from build123d import *

# Parameters (mm, degrees)
SKETCH_1_W             = 35.69
SKETCH_1_H             = 89.14
SM_BASE_FLANGE_1_DEPTH = 2.85
OTHER_START            = -17.845
OTHER_1_DEPTH          = 35.69
OTHER_1_2_DEPTH        = 35.69
SKETCH_7_R             = 14.0825
SKETCH_7_R_2           = 1.845
CUT_EXTRUDE_1_DEPTH    = 10
CHAMFER_1_SIZE         = 3
SKETCH_8_R             = 2.795
CUT_EXTRUDE_2_DEPTH    = 10


# Read off the part's stored shape, not the designer's step: Нарисованный сгиб1
# Sheet-metal steps are written as plain solids
with BuildPart() as part:
    # Sketch 1 → Базовая кромка1 (new body)
    with BuildSketch(Plane(origin=(0, 0, 0), x_dir=(1, 0, 0), z_dir=(0, 1, 0))):
        Rectangle(SKETCH_1_W, SKETCH_1_H)
    extrude(amount=-SM_BASE_FLANGE_1_DEPTH)

    # Other 1 outline → Other 1 (cut)
    with BuildSketch(Plane.YZ.offset(OTHER_START)):
        with BuildLine():
            Line((0, -44.57), (0, 6.169199698))
            ThreePointArc((0, 6.169199698), (-2.096002789, 8.605700079), (-2.85, 11.73))
            Line((-2.85, 11.73), (-2.85, -44.57))
            Line((-2.85, -44.57), (0, -44.57))
        make_face()
    extrude(amount=OTHER_1_DEPTH, mode=Mode.SUBTRACT)

    # Other 1 2 outline → Other 1 2 (add)
    with BuildSketch(Plane.YZ.offset(OTHER_START)):
        with BuildLine():
            Line((51.778429927, 7.73), (4, 7.73))
            ThreePointArc((4, 7.73), (1.171572875, 8.901572875), (0, 11.73))
            Line((0, 11.73), (0, 6.169199698))
            ThreePointArc((0, 6.169199698), (1.898688751, 5.210261429), (4, 4.88))
            Line((4, 4.88), (51.778429927, 4.88))
            Line((51.778429927, 4.88), (51.778429927, 7.73))
        make_face()
    extrude(amount=OTHER_1_2_DEPTH)

    # Эскиз7 → Вырез-Вытянуть1 (cut)
    with BuildSketch(Plane.XY.offset(7.73)):
        with Locations((0, 33.778429927)):
            Circle(SKETCH_7_R)
        with Locations((13, 46.778429927)):
            Circle(SKETCH_7_R_2)
        with Locations(Location((-13, 46.778429927, 0), (0, 0, 90))):
            Circle(SKETCH_7_R_2)
        with Locations((-13, 20.778429927)):
            Circle(SKETCH_7_R_2)
        with Locations(Location((13, 20.778429927, 0), (0, 0, 90))):
            Circle(SKETCH_7_R_2)
    extrude(amount=-CUT_EXTRUDE_1_DEPTH, mode=Mode.SUBTRACT)

    # Фаска1
    chamfer_1_edges = [part.edges().sort_by_distance(p)[0] for p in [
        (17.845, -1.425, 44.57),
        (-17.845, -1.425, 44.57),
        (-17.845, 51.778429927, 6.305),
        (17.845, 51.778429927, 6.305),
    ]]
    chamfer(chamfer_1_edges, length=CHAMFER_1_SIZE)

    # Эскиз8 → Вырез-Вытянуть2 (cut)
    with BuildSketch(Plane(origin=(0, 0, 0), x_dir=(1, 0, 0), z_dir=(0, 1, 0))):
        with Locations(Location((-10, -29.57, 0), (0, 0, 270))):
            Circle(SKETCH_8_R)
        with Locations(Location((10, -29.57, 0), (0, 0, 90))):
            Circle(SKETCH_8_R)
    extrude(amount=-CUT_EXTRUDE_2_DEPTH, mode=Mode.SUBTRACT)


solid = part.part
Build history of the part. All positions in model axes, mm. A direction names the side the tool comes from. Round coordinates to 2 decimals unless told otherwise and drop trailing zeros. Write each loop counter-clockwise with the first axis right and the second up, starting at its lowest first coordinate (ties: lowest second). Pieces come first, ordered by that corner, then holes. Notation, with made-up numbers: (13, -16.5) - (33, -16.5) arc R21 ccw to (33, 1.5) - close; hole circle Ø7 at (38.25, 56.25). An arc over 180 degrees is marked (long way). One line per question, with ' | ' between items.
1. Drop a flat-ended pin along its axis: pin 1 Ø2 at (x, y) = (-11, 19) entering from +Z. Give the stop position or say it passes through.
Results are:
pin 1: z = 7.73
2. Band-saw the part on D-D, the plane x = 9. Write the cut outline in (y, z).
Results are:
outline: (-2.85, 11.73) arc R6.85 ccw to (4, 4.88) - (22.95, 4.88) - (22.95, 7.73) - (4, 7.73) arc R4 cw to (0, 11.73) - (0, 26.96) - (-2.85, 26.96) - close; (-2.85, 32.18) - (0, 32.18) - (0, 44.57) - (-2.85, 44.57) - close; (44.61, 4.88) - (51.78, 4.88) - (51.78, 7.73) - (44.61, 7.73) - close
3. Mould opens along X. For faces 3 (the face through (17.845, 11, 7)), 4 (the face through (-12.15, 19.14, 6.32)), 5 (the face through (-16.324, -1.405, 43.091)), 6 (the face through (0, 17, 4.88)) say: released by +X, released by -X, zero draft, split by the parting line, or undercut.
Results are:
face 3: released by +X | face 4: undercut | face 5: released by -X | face 6: zero draft
4. Band-saw the part on A-A, the plane z = 29.57. Write the cut outline in (x, y) (3 decimals).
Results are:
outline: (-17.845, -2.85) - (-12.795, -2.85) - (-12.795, 0) - (-17.845, 0) - close; (-7.205, -2.85) - (7.205, -2.85) - (7.205, 0) - (-7.205, 0) - close; (12.795, -2.85) - (17.845, -2.85) - (17.845, 0) - (12.795, 0) - close
5. Band-saw the part on C-C, the plane y = 32.5. Write the cut outline in (x, z) (3 decimals), and give its area (3 significant figures).
Results are:
outline: (-17.845, 4.88) - (-14.024, 4.88) - (-14.024, 7.73) - (-17.845, 7.73) - close; (14.024, 4.88) - (17.845, 4.88) - (17.845, 7.73) - (14.024, 7.73) - close | area: 21.8 mm^2
6. Band-saw the part on B-B, the plane x = 0. Write the cut outline in (y, z), and give its area (3 significant figures).
Results are:
outline: (-2.85, 11.73) arc R6.85 ccw to (4, 4.88) - (19.7, 4.88) - (19.7, 7.73) - (4, 7.73) arc R4 cw to (0, 11.73) - (0, 44.57) - (-2.85, 44.57) - close; (47.86, 4.88) - (51.78, 4.88) - (51.78, 7.73) - (47.86, 7.73) - close | area: 174 mm^2
7. Drill centre lines: line 1 along X through (y, z) = (-0.7, 29.57) (3 decimals); line 2 along Z through (x, y) = (14.5, 32.5); line 3 along Y through (x, z) = (13, 6). Where is each one in solid material? Low to high. Write a range as from..to.
Results are:
line 1: -17.845..-12.795, -7.205..7.205, 12.795..17.845 | line 2: 4.88..7.73 | line 3: 0.25..18.93, 22.62..28.36, 39.19..44.93, 48.62..51.78
8. Tool access for faces 1 (the face through (0, 0, 28)), 2 (the face through (0, -1, 44.57)): list every direction of +Z, -Z, +X, -X, +Y, -Y with a clear straight run to the whole face (end or side of a thin tool).
Results are:
face 1: +Z, +X, -X, +Y | face 2: +Z, +X, -X, +Y, -Y
